```python
from build123d import *

# Parameters (mm, degrees)
BASE_FLANGE1_DEPTH   = 997
CUT_EXTRUDE1_DEPTH   = 10
SKETCH5_R            = 4
CUT_EXTRUDE2_DEPTH   = 10
CUT_EXTRUDE4_DEPTH   = 10
LPATTERN1_COUNT      = 3
LPATTERN1_PITCH      = 375
LPATTERN1_COUNT_DIR2 = 2
LPATTERN1_PITCH_DIR2 = 564.02
CHAMFER1_SIZE        = 4


# Sheet-metal steps are written as plain solids
with BuildPart() as part:
    # Sketch1 → Base-Flange1 (new body)
    with BuildSketch(Plane(origin=(0, 0, 0), x_dir=(1, 0, 0), z_dir=(0, 1, 0))):
        with BuildLine():
            Line((116.152236891, -603), (297.071067812, -422.08116908))
            ThreePointArc((297.071067812, -422.08116908), (299.238795325, -418.836935591), (300, -415.010101268))
            Line((300, -415.010101268), (300, 211.010101268))
            ThreePointArc((300, 211.010101268), (299.238795325, 214.836935591), (297.071067812, 218.08116908))
            Line((297.071067812, 218.08116908), (119.08116908, 396.071067812))
            ThreePointArc((119.08116908, 396.071067812), (115.836935591, 398.238795325), (112.010101268, 399))
            Line((112.010101268, 399), (-516, 399))
            Line((-516, 399), (-516, 395))
            Line((-516, 395), (112.010101268, 395))
            ThreePointArc((112.010101268, 395), (114.306201862, 394.543277195), (116.252741955, 393.242640687))
            Line((116.252741955, 393.242640687), (294.242640687, 215.252741955))
            ThreePointArc((294.242640687, 215.252741955), (295.543277195, 213.306201862), (296, 211.010101268))
            Line((296, 211.010101268), (296, -415.010101268))
            ThreePointArc((296, -415.010101268), (295.543277195, -417.306201862), (294.242640687, -419.252741955))
            Line((294.242640687, -419.252741955), (113.323809767, -600.171572875))
            Line((113.323809767, -600.171572875), (116.152236891, -603))
        make_face()
    extrude(amount=BASE_FLANGE1_DEPTH)

    # Sketch2 → Cut-Extrude1 (cut)
    with BuildSketch(Plane(origin=(257.576118446, 0, -257.576118446), x_dir=(-0.7071067811865485, 0, -0.7071067811865466), z_dir=(0.7071067811865466, 0, -0.7071067811865485))):
        with BuildLine():
            Line((170.145706961, 234), (170.145706961, 134))
            ThreePointArc((170.145706961, 134), (70.145706961, 34), (-29.854293039, 134))
            Line((-29.854293039, 134), (-29.854293039, 234))
            ThreePointArc((-29.854293039, 234), (70.145706961, 334), (170.145706961, 234))
        make_face()
    extrude(amount=-CUT_EXTRUDE1_DEPTH, mode=Mode.SUBTRACT)

    # Sketch5 → Cut-Extrude2 (cut)
    with BuildSketch(Plane.ZY.offset(-296)):
        with Locations((384.010101268, 873.5)):
            Circle(SKETCH5_R)
    cut_extrude2 = extrude(amount=-CUT_EXTRUDE2_DEPTH, mode=Mode.SUBTRACT)

    # Sketch7 → Cut-Extrude4 (cut)
    with BuildSketch(Plane(origin=(359.576118446, 0, 359.576118446), x_dir=(0.7071067811865416, 0, -0.7071067811865536), z_dir=(0.7071067811865536, 0, 0.7071067811865416))):
        with BuildLine():
            Line((-114.395490323, 234), (-114.395490323, 134))
            ThreePointArc((-114.395490323, 134), (-214.395490323, 34), (-314.395490323, 134))
            Line((-314.395490323, 134), (-314.395490323, 234))
            ThreePointArc((-314.395490323, 234), (-214.395490323, 334), (-114.395490323, 234))
        make_face()
    extrude(amount=-CUT_EXTRUDE4_DEPTH, mode=Mode.SUBTRACT)

    # LPattern1: Cut-Extrude2 3 × 2
    with Locations(*[(0, -i * LPATTERN1_PITCH, -j * LPATTERN1_PITCH_DIR2) for i in range(LPATTERN1_COUNT) for j in range(LPATTERN1_COUNT_DIR2) if (i, j) != (0, 0)]):
        add(cut_extrude2, mode=Mode.SUBTRACT)

    # Chamfer1
    chamfer1_edges = [part.edges().sort_by_distance(p)[0] for p in [
        (116.152236891, 498.5, 603),
        (-516, 498.5, -399),
    ]]
    chamfer(chamfer1_edges, length=CHAMFER1_SIZE - 0.0001)  # a hair under: the kernel refuses the full size


solid = part.part
```
Geometry check sheet. Reference: the model listing, model coordinates, mm. A direction names the side the tool comes from. Round coordinates to 2 decimals unless told otherwise and drop trailing zeros. Order: outer loops, then holes, each group sorted by start corner. A loop starts at its lowest first (then second) coordinate and runs counter-clockwise, first axis right, second up. Notation, with made-up numbers: (12, 40.5) - (39, 40.5) arc R23 ccw to (39, 75.5) - close; hole circle Ø3 at (72.25, 67). An arc over 180 degrees is marked (long way). Use a Markdown table: item, result. Add a question column.
(1) Sectioned sample at D-D, the plane x = 63. Enter the section's corners in (y, z), and give its area (3 significant figures).
(2) Sectioned sample at B-B, the plane z = -5. Enter the section's corners in (x, y).
(3) Sectioned sample at C-C, the plane x = 183. Count the separate pieces of the cut face and the enclosed holes in it, and give its area (3 significant figures).
(4) Material ranges on line 1 along Z through (x, y) = (297.05, 873.5); line 2 along Z through (x, y) = (297, 123); line 3 along X through (y, z) = (366.5, -41), recorded low to high. Write a range as [from, to].
(5) Depth check by flat-ended pin: pin 1 (12 mm diameter, centred on y = 197, z = -225.5, fed in from -X); pin 2 (6 mm diameter, centred on y = 321.5, z = 377, fed in from -X); pin 3 (3 mm diameter, centred on y = 294.5, z = -245.5, fed in from +X). Enter the tip coordinate at first touch or a pass-through.
(6) Tool access check on faces 5 (the cylindrical face through (205.026, 333.976, 511.337)), 6 (the flat face through (-206, 492, -395)), 7 (the flat face through (205.05, 602.299, 508.446)). Record the directions out of +Z, -Z, +X, -X, +Y, -Y that give a thin tool (end or side, any length) a straight path to the whole face; none if there is none.
(7) Release check for a two-part mould opening along Z. For faces 1 (the flat face through (300, 492, 106)), 2 (the flat face through (209.32, 602.3, -305.83)), 3 (the flat face through (296, 492, 98)), 4 (the flat face through (206.78, 602.3, 512.37)) record: pulls with the +Z half, pulls with the -Z half, needs draft (parallel to the pull), parting line crosses it, or undercut.
Answers below:
| question | item | result |
|---|---|---|
| 1 | outline | (0, -399) - (997, -399) - (997, -395) - (0, -395) - close |
| 1 | area | 3,990 mm² |
| 2 | outline | (296, 0) - (300, 0) - (300, 997) - (296, 997) - close |
| 3 | separate pieces | 4 |
| 3 | enclosed holes | 0 |
| 3 | area | 8,020 mm² |
| 4 | line 1 | [-218.1, -184.01], [-176.01, 380.01], [388.01, 422.1] |
| 4 | line 2 | [-218.15, -183.98], [-176.04, 380.04], [387.98, 422.15] |
| 4 | line 3 | [296, 300] |
| 5 | pin 1 | x = 278 |
| 5 | pin 2 | x = 296 |
| 5 | pin 3 | x = 271.15 |
| 6 | face 5 | none |
| 6 | face 6 | +Z, -X, +Y, -Y |
| 6 | face 7 | -X, +Y, -Y |
| 7 | face 1 | needs draft |
| 7 | face 2 | pulls with the -Z half |
| 7 | face 3 | undercut |
| 7 | face 4 | pulls with the +Z half |
